```python
from build123d import *

# Parameters (mm, degrees)
BOSS_EXTRUDE1_DEPTH   = 6
F_6_CLEARANCE_HOLE1_D = 3.7973
CUT_EXTRUDE1_REACH    = 34.362
FILLET1_R             = 2.61
M2_CLEARANCE_HOLE1_D  = 2.4


with BuildPart() as part:
    # Sketch1 → Boss-Extrude1 (new body)
    with BuildSketch(Plane.XY):
        with BuildLine():
            ThreePointArc((-8, 6.7), (-5.656854249, 12.356854249), (0, 14.7))
            Line((0, 14.7), (20.2, 14.7))
            ThreePointArc((20.2, 14.7), (25.856854249, 12.356854249), (28.2, 6.7))
            Line((28.2, 6.7), (28.2, 0))
            Line((28.2, 0), (20.2, 0))
            Line((20.2, 0), (20.2, 6.7))
            Line((20.2, 6.7), (0, 6.7))
            Line((0, 6.7), (0, 0))
            Line((0, 0), (-8, 0))
            Line((-8, 0), (-8, 6.7))
        make_face()
    extrude(amount=BOSS_EXTRUDE1_DEPTH)

    # #6 Clearance Hole1 (through all)
    with Locations(Plane.XY.offset(6)):
        with Locations((10.1, 10.7)):
            Hole(F_6_CLEARANCE_HOLE1_D / 2)

    # Sketch5 → Cut-Extrude1 (cut, up to next)
    with BuildSketch(Plane.XY.offset(6), mode=Mode.PRIVATE) as cut_extrude1_sk1:
        with BuildLine():
            Line((7, 14.7), (3, 14.7))
            Line((3, 14.7), (3, 12.093133814))
            Line((3, 12.093133814), (7, 12.093133814))
            ThreePointArc((7, 12.093133814), (10.1, 14.09865), (13.2, 12.093133814))
            Line((13.2, 12.093133814), (17.2, 12.093133814))
            Line((17.2, 12.093133814), (17.2, 14.7))
            Line((17.2, 14.7), (13.2, 14.7))
            Line((13.2, 14.7), (7, 14.7))
        make_face()
    cut_extrude1_tool1 = extrude(cut_extrude1_sk1.sketch, amount=-CUT_EXTRUDE1_REACH, mode=Mode.PRIVATE) & part.part
    add(cut_extrude1_tool1.solids().sort_by_distance((10.1, 14.243023, 6))[0], mode=Mode.SUBTRACT)

    # Fillet1
    # the kernel refuses this fillet: 2.61 mm, written as the material it takes off along each edge
    with BuildSketch(Plane(origin=(17.2, 14.7, 12.524995297), x_dir=(1, 0, 0), z_dir=(0, 0, -1))) as fillet1_piece_1:
        with BuildLine():
            CenterArc((2.609998119, 2.61), FILLET1_R, 180.068794764, 89.931205236)
            Line((0, 2.606866186), (-0.052199962, 2.60680351))
            Line((-0.052199962, 2.60680351), (-0.0522, 0))
            Line((-0.0522, 0), (0, -0.0522))
            Line((0, -0.0522), (2.609998119, -0.0522))
            Line((2.609998119, -0.0522), (2.609998119, 0))
        make_face()
    extrude(amount=19.049990593, mode=Mode.SUBTRACT)
    with BuildSketch(Plane(origin=(3, 14.7, 12.524995297), x_dir=(-1, 0, 0), z_dir=(0, 0, -1))) as fillet1_piece_2:
        with BuildLine():
            CenterArc((2.609998119, -2.61), FILLET1_R, 90, 89.931205236)
            Line((0, -2.606866186), (-0.052199962, -2.60680351))
            Line((-0.052199962, -2.60680351), (-0.0522, 0))
            Line((-0.0522, 0), (0, 0.0522))
            Line((0, 0.0522), (2.609998119, 0.0522))
            Line((2.609998119, 0.0522), (2.609998119, 0))
        make_face()
    extrude(amount=19.049990593, mode=Mode.SUBTRACT)

    # M2 Clearance Hole1 (through all)
    with Locations(Plane(origin=(0, 12.093133814, 0), x_dir=(1, 0, 0), z_dir=(0, 1, 0))):
        with Locations((5, -3), (15.2, -3)):
            Hole(M2_CLEARANCE_HOLE1_D / 2)


solid = part.part
```
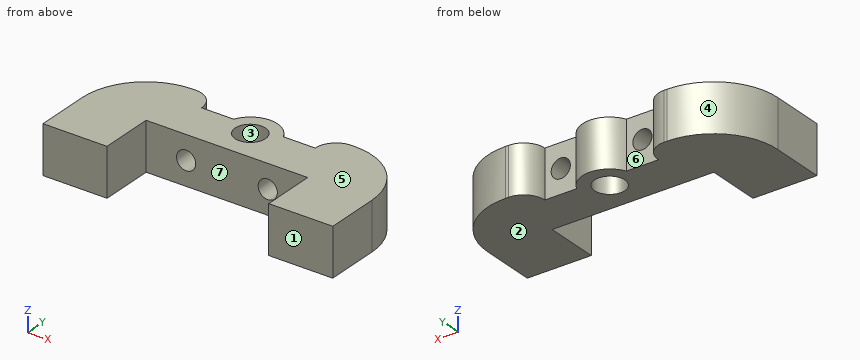
CAD build for the part. Positions are in the model's coordinates, mm. Face numbers are marked on the shaded views. A direction names the side the tool comes from. Round coordinates to 2 decimals unless told otherwise and drop trailing zeros. Order: outer loops, then holes, each group sorted by start corner. A loop starts at its lowest first (then second) coordinate and runs counter-clockwise, first axis right, second up. Notation, with made-up numbers: (13.5, 83.5) - (36.5, 83.5) arc R28 ccw to (36.5, 104.5) - close; hole circle Ø11 at (57.25, -4). An arc over 180 degrees is marked (long way). Use CSV: the item, a comma, the result in double quotes. Start each with the question number.
1) Pin check, flat tips, straight feed: pin 1 Ø2 at (x, z) = (16, 4.5) entering from +Y; pin 2 Ø3 at (x, z) = (15.2, 3) entering from -Y; pin 3 Ø1 at (y, z) = (9.5, 2.5) entering from -X; pin 4 Ø4 at (x, y) = (3.5, 4) entering from -Z. Stop position of each tip, or through.
2) Saw through at D-D (y = 10.7). List the corners of the cut face in (x, z).
3) Wall check: L1, parallel to X at y = 6, z = 4.55; L2, parallel to Z at x = 5, y = 8.5; L3, parallel to X at y = 7.5, z = 4.05. Give the ranges that are in metal, low to high. Write a range as [from, to].
4) Saw through at C-C (x = 5). List the corners of the cut face in (y, z).
5) Saw through at A-A (z = 3). List the corners of the cut face in (x, y), and give its area (3 significant figures).
6) Saw through at B-B (y = 3). List the corners of the cut face in (x, z), and give its area (3 significant figures).
7) Tool access for the marked faces 5, 6 and 7: list every direction of +Z, -Z, +X, -X, +Y, -Y with a clear straight run to the whole face (end or side of a thin tool).
8) Two-plate mould, pull along Y, no slides. Class the marked faces 1, 2, 3 and 4: pulls with the +Y half, pulls with the -Y half, needs draft (parallel to the pull), parting line crosses it, or undercut.
Values follow:
1,pin 1,"stops at y = 12.09"
1,pin 2,"stops at y = 6.7"
1,pin 3,"stops at x = -7.66"
1,pin 4,"passes through"
2,outline,"(-6.93, 0) - (8.2, 0) - (8.2, 6) - (-6.93, 6) - close; (12, 0) - (27.13, 0) - (27.13, 6) - (12, 6) - close; hole circle Ø2.4 at (5, 3); hole circle Ø2.4 at (15.2, 3)"
3,L1,"x = [-8, 0], [20.2, 28.2]"
3,L2,"z = [0, 1.8], [4.2, 6]"
3,L3,"x = [-7.96, 4.42], [5.58, 14.62], [15.78, 28.16]"
4,outline,"(6.7, 0) - (12.09, 0) - (12.09, 1.8) - (6.7, 1.8) - close; (6.7, 4.2) - (12.09, 4.2) - (12.09, 6) - (6.7, 6) - close"
5,outline,"(-8, 0) - (0, 0) - (0, 6.7) - (3.8, 6.7) - (3.8, 12.09) - (3, 12.09) arc R2.61 ccw to (0.39, 14.7) - (0, 14.7) arc R8 ccw to (-8, 6.7) - close; (6.2, 6.7) - (14, 6.7) - (14, 12.09) - (13.2, 12.09) arc R3.4 ccw to (7, 12.09) - (6.2, 12.09) - close; (16.4, 6.7) - (20.2, 6.7) - (20.2, 0) - (28.2, 0) - (28.2, 6.7) arc R8 ccw to (20.2, 14.7) - (19.81, 14.7) arc R2.61 ccw to (17.2, 12.09) - (16.4, 12.09) - close; hole circle Ø3.8 at (10.1, 10.7)"
5,area,"301 mm2"
6,outline,"(-8, 0) - (0, 0) - (0, 6) - (-8, 6) - close; (20.2, 0) - (28.2, 0) - (28.2, 6) - (20.2, 6) - close"
6,area,"96.0 mm2"
7,face 5,"+Z, +X, -X, +Y, -Y"
7,face 6,"+Z, -Z, +Y"
7,face 7,"+Z, -Z, -Y"
8,face 1,"pulls with the -Y half"
8,face 2,"needs draft"
8,face 3,"undercut"
8,face 4,"pulls with the +Y half"
